The figure shows three views and two pictorial views of one solid part (mm, origin at its lowest corner). Answer the questions. Coordinates: 2 decimals unless noted, no trailing zeros. Write each loop counter-clockwise with the first axis right and the second up, starting at its lowest first coordinate (ties: lowest second). Pieces come first, ordered by that corner, then holes.
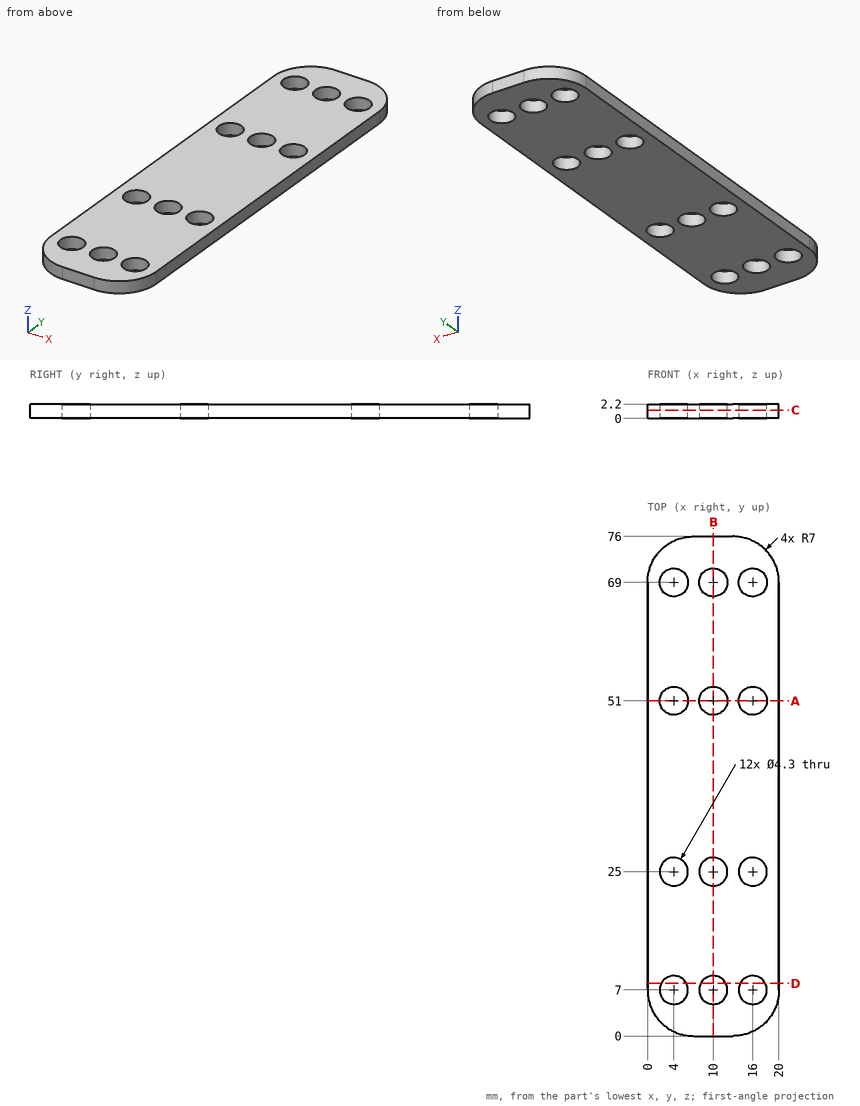
1. Section A-A on y = 51 is taken. Give the vertices of the cut face in (x, z), then the cut area to 3 significant figures.
Results found:
outline: (0, 0) - (1.85, 0) - (1.85, 2.2) - (0, 2.2) - close; (6.15, 0) - (7.85, 0) - (7.85, 2.2) - (6.15, 2.2) - close; (12.15, 0) - (13.85, 0) - (13.85, 2.2) - (12.15, 2.2) - close; (18.15, 0) - (20, 0) - (20, 2.2) - (18.15, 2.2) - close
area: 15.6 mm2
2. Section C-C on z = 1.25 is taken. State how many separate pieces and enclosed holes the cut face has, then the cut area to 3 significant figures.
Results found:
separate pieces: 1
enclosed holes: 12
area: 1,300 mm2
3. Section B-B on x = 10 is taken. Give the vertices of the cut face in (y, z).
Results found:
outline: (0, 0) - (4.85, 0) - (4.85, 2.2) - (0, 2.2) - close; (9.15, 0) - (22.85, 0) - (22.85, 2.2) - (9.15, 2.2) - close; (27.15, 0) - (48.85, 0) - (48.85, 2.2) - (27.15, 2.2) - close; (53.15, 0) - (66.85, 0) - (66.85, 2.2) - (53.15, 2.2) - close; (71.15, 0) - (76, 0) - (76, 2.2) - (71.15, 2.2) - close
4. Find the intervals of material crossed by L1, parallel to X at y = 51, z = 0.65; L2, parallel to Y at x = 10, z = 1.7; L3, parallel to Y at x = 16, z = 0.6, in increasing order.
Results found:
L1: x = 0 to 1.85, 6.15 to 7.85, 12.15 to 13.85, 18.15 to 20
L2: y = 0 to 4.85, 9.15 to 22.85, 27.15 to 48.85, 53.15 to 66.85, 71.15 to 76
L3: y = 0.68 to 4.85, 9.15 to 22.85, 27.15 to 48.85, 53.15 to 66.85, 71.15 to 75.32
5. Section D-D on y = 8 is taken. Give the vertices of the cut face in (x, z), then the cut area to 3 significant figures.
Results found:
outline: (0, 0) - (2.1, 0) - (2.1, 2.2) - (0, 2.2) - close; (5.9, 0) - (8.1, 0) - (8.1, 2.2) - (5.9, 2.2) - close; (11.9, 0) - (14.1, 0) - (14.1, 2.2) - (11.9, 2.2) - close; (17.9, 0) - (20, 0) - (20, 2.2) - (17.9, 2.2) - close
area: 18.9 mm2
